```python
from build123d import *

# Parameters (mm, degrees)
SKETCH_1_W             = 60
SKETCH_1_H             = 124
EXTRUDE_1_DEPTH        = 3
EXTRUDE_2_DEPTH        = 3
SKETCH_3_W             = 136
SKETCH_3_H             = 57.699964
EXTRUDE_3_DEPTH        = 3
CUT_EXTRUDE_1_DEPTH    = 3
SKETCH_5_W             = 22
SKETCH_5_H             = 12
CUT_EXTRUDE_2_DEPTH    = 10
SKETCH_6_R             = 1.275
CUT_EXTRUDE_3_DEPTH    = 10
PATTERN_LINEAR_1_COUNT = 2
PATTERN_LINEAR_1_PITCH = 7.5
PATTERN_LINEAR_2_COUNT = 2
PATTERN_LINEAR_2_PITCH = 7.5
SKETCH_7_R             = 1.525
CUT_EXTRUDE_4_DEPTH    = 10
FILLET_1_R             = 2
SKETCH_8_W             = 21
SKETCH_8_H             = 41.4
CUT_EXTRUDE_5_DEPTH    = 22
FILLET_2_R             = 2
SKETCH_10_W            = 80
SKETCH_10_H            = 20.2
CUT_EXTRUDE_6_DEPTH    = 3
FILLET_3_R             = 2
CUT_EXTRUDE_7_DEPTH    = 3
EXTRUDE_5_DEPTH        = 3
CUT_EXTRUDE_START      = -22
SKETCH_13_R            = 5.6
CUT_EXTRUDE_8_DEPTH    = 115.070625066
FILLET_4_R             = 2


with BuildPart() as part:
    # 草图1 → 凸台-拉伸1 (new body)
    with BuildSketch(Plane.XY):
        Rectangle(SKETCH_1_W, SKETCH_1_H)
    extrude(amount=EXTRUDE_1_DEPTH)

    # 草图2 → 凸台-拉伸2 (add)
    with BuildSketch(Plane(origin=(0, 0, 0), x_dir=(-1, 0, 0), z_dir=(0, 0, -1))):
        Polygon((-66.648513504, -4.300036), (66.648513504, -4.300036), (30, 36.746299124), (-30, 36.746299124), align=None)
    extrude(amount=-EXTRUDE_2_DEPTH)

    # 草图3 → 凸台-拉伸3 (add)
    with BuildSketch(Plane.XY.offset(3)):
        with Locations((0, -33.150018)):
            Rectangle(SKETCH_3_W, SKETCH_3_H)
    extrude(amount=-EXTRUDE_3_DEPTH)

    # 草图4 → 切除-拉伸1 (cut)
    with BuildSketch(Plane.XY.offset(3)):
        Polygon((68, -4.300036), (68, -5.813700876), (66.648513504, -4.300036), align=None)
        Polygon((-66.648513504, -4.300036), (-68, -4.300036), (-68, -5.813700876), align=None)
    extrude(amount=-CUT_EXTRUDE_1_DEPTH, mode=Mode.SUBTRACT)

    # 草图5 → 切除-拉伸2 (cut)
    with BuildSketch(Plane(origin=(0, 0, 0), x_dir=(-1, 0, 0), z_dir=(0, 0, -1))):
        with Locations((-57, -56)):
            Rectangle(SKETCH_5_W, SKETCH_5_H)
    cut_extrude_2 = extrude(amount=-CUT_EXTRUDE_2_DEPTH, mode=Mode.SUBTRACT)

    # 镜向1: 切除-拉伸2 across plane
    add(cut_extrude_2.mirror(Plane(origin=(0, 0, 0), x_dir=(0, 0, 1), z_dir=(1, 0, 0))), mode=Mode.SUBTRACT)

    # 草图6 → 切除-拉伸3 (cut)
    with BuildSketch(Plane(origin=(0, 0, 0), x_dir=(-1, 0, 0), z_dir=(0, 0, -1))):
        with Locations((-27, 50.7)):
            Circle(SKETCH_6_R)
        with Locations((27, 50.7)):
            Circle(SKETCH_6_R)
        with Locations((27, -21.3)):
            Circle(SKETCH_6_R)
        with Locations((-27, -21.3)):
            Circle(SKETCH_6_R)
    cut_extrude_3 = extrude(amount=-CUT_EXTRUDE_3_DEPTH, mode=Mode.SUBTRACT)

    # 阵列(线性)1: 切除-拉伸3 ×2
    with Locations(*[(0, i * PATTERN_LINEAR_1_PITCH, 0) for i in range(1, PATTERN_LINEAR_1_COUNT)]):
        add(cut_extrude_3, mode=Mode.SUBTRACT)

    # 阵列(线性)2: 切除-拉伸3 ×2
    with Locations(*[(0, -i * PATTERN_LINEAR_2_PITCH, 0) for i in range(1, PATTERN_LINEAR_2_COUNT)]):
        add(cut_extrude_3, mode=Mode.SUBTRACT)

    # 草图7 → 切除-拉伸4 (cut)
    with BuildSketch(Plane(origin=(0, 0, 0), x_dir=(-1, 0, 0), z_dir=(0, 0, -1))):
        with Locations((65, -45)):
            Circle(SKETCH_7_R)
        with Locations((65, -25)):
            Circle(SKETCH_7_R)
        with Locations((41.234077164, 19.659734849)):
            Circle(SKETCH_7_R)
        with Locations((54.554392551, 4.740981616)):
            Circle(SKETCH_7_R)
    cut_extrude_4 = extrude(amount=-CUT_EXTRUDE_4_DEPTH, mode=Mode.SUBTRACT)

    # 镜向2: 切除-拉伸4 across plane
    add(cut_extrude_4.mirror(Plane(origin=(0, 0, 0), x_dir=(0, 0, 1), z_dir=(1, 0, 0))), mode=Mode.SUBTRACT)

    # 圆角1
    fillet_1_edges = [part.edges().sort_by_distance(p)[0] for p in [
        (-68, -50, 1.5),
        (-46, -62, 1.5),
        (-46, -50, 1.5),
        (-30, 36.746299124, 1.5),
        (30, 36.746299124, 1.5),
        (68, -5.813700876, 1.5),
        (-68, -5.813700876, 1.5),
        (-30, 62, 1.5),
        (30, 62, 1.5),
        (68, -50, 1.5),
        (46, -50, 1.5),
        (46, -62, 1.5),
    ]]
    fillet(fillet_1_edges, radius=FILLET_1_R)

    # 草图8 → 切除-拉伸5 (cut)
    with BuildSketch(Plane(origin=(0, 0, 0), x_dir=(-1, 0, 0), z_dir=(0, 0, -1))):
        with Locations((-13.5, -11.1)):
            Rectangle(SKETCH_8_W, SKETCH_8_H)
        with Locations((13.5, -11.1)):
            Rectangle(SKETCH_8_W, SKETCH_8_H)
        with Locations((13.5, 36.3)):
            Rectangle(SKETCH_8_W, SKETCH_8_H)
        with Locations((-13.5, 36.3)):
            Rectangle(SKETCH_8_W, SKETCH_8_H)
    extrude(amount=-CUT_EXTRUDE_5_DEPTH, mode=Mode.SUBTRACT)

    # 圆角2
    fillet_2_edges = [part.edges().sort_by_distance(p)[0] for p in [
        (24, 15.6, 1.5),
        (24, 57, 1.5),
        (3, 57, 1.5),
        (3, 15.6, 1.5),
        (-3, 57, 1.5),
        (-24, 57, 1.5),
        (-24, 15.6, 1.5),
        (-3, 15.6, 1.5),
        (-3, 9.6, 1.5),
        (-24, 9.6, 1.5),
        (-24, -31.8, 1.5),
        (-3, -31.8, 1.5),
        (3, 9.6, 1.5),
        (3, -31.8, 1.5),
        (24, -31.8, 1.5),
        (24, 9.6, 1.5),
    ]]
    fillet(fillet_2_edges, radius=FILLET_2_R)

    # 草图10 → 切除-拉伸6 (cut)
    with BuildSketch(Plane(origin=(0, 0, 0), x_dir=(-1, 0, 0), z_dir=(0, 0, -1))):
        with Locations((0, -46.9)):
            Rectangle(SKETCH_10_W, SKETCH_10_H)
    extrude(amount=-CUT_EXTRUDE_6_DEPTH, mode=Mode.SUBTRACT)

    # 圆角3
    fillet_3_edges = [part.edges().sort_by_distance(p)[0] for p in [
        (-40, -36.8, 1.5),
        (-40, -57, 1.5),
        (40, -57, 1.5),
        (40, -36.8, 1.5),
    ]]
    fillet(fillet_3_edges, radius=FILLET_3_R)

    # 草图11 → 切除-拉伸7 (cut)
    with BuildSketch(Plane.XY.offset(3)):
        Polygon((-31, 26.617503422), (-59, -4.742496578), (-59, -30.8), (-31, -30.8), align=None)
    cut_extrude_7 = extrude(amount=-CUT_EXTRUDE_7_DEPTH, mode=Mode.SUBTRACT)

    # 镜向3: 切除-拉伸7 across plane
    add(cut_extrude_7.mirror(Plane(origin=(0, 0, 0), x_dir=(0, 0, 1), z_dir=(1, 0, 0))), mode=Mode.SUBTRACT)

    # 草图12 → 凸台-拉伸5 (add)
    with BuildSketch(Plane(origin=(0, 0, 0), x_dir=(-1, 0, 0), z_dir=(0, 0, -1))):
        with BuildLine():
            Line((-59, -6.742496578), (-31, -6.742496578))
            ThreePointArc((-31, -6.742496578), (-29, -4.742496578), (-31, -2.742496578))
            Line((-31, -2.742496578), (-59, -2.742496578))
            ThreePointArc((-59, -2.742496578), (-61, -4.742496578), (-59, -6.742496578))
        make_face()
    extrude_5 = extrude(amount=-EXTRUDE_5_DEPTH)

    # 镜向4: 凸台-拉伸5 across plane
    add(extrude_5.mirror(Plane(origin=(0, 0, 0), x_dir=(0, 0, 1), z_dir=(1, 0, 0))))

    # 草图13 → 切除-拉伸8 (cut)
    with BuildSketch(Plane(origin=(0, 0, 0), x_dir=(-1, 0, 0), z_dir=(0, 0, -1)).offset(CUT_EXTRUDE_START)):
        with Locations(Location((53.4, -40.4, 0), (0, 0, 180))):
            Circle(SKETCH_13_R)
    cut_extrude_8 = extrude(amount=CUT_EXTRUDE_8_DEPTH, mode=Mode.SUBTRACT)

    # 镜向5: 切除-拉伸8 across plane
    add(cut_extrude_8.mirror(Plane(origin=(0, 0, 0), x_dir=(0, 0, 1), z_dir=(1, 0, 0))), mode=Mode.SUBTRACT)

    # 圆角4
    fillet_4_edges = [part.edges().sort_by_distance(p)[0] for p in [
        (-59, -30.8, 1.5),
        (-31, -30.8, 1.5),
        (-31, 26.617503422, 1.5),
        (31, -30.8, 1.5),
        (31, 26.617503422, 1.5),
        (59, -30.8, 1.5),
        (57.214285714, -2.742496578, 1.5),
        (59, -6.742496578, 1.5),
        (31, -2.742496578, 1.5),
        (31, -6.742496578, 1.5),
        (-57.214285714, -2.742496578, 1.5),
        (-31, -2.742496578, 1.5),
        (-31, -6.742496578, 1.5),
        (-59, -6.742496578, 1.5),
    ]]
    fillet(fillet_4_edges, radius=FILLET_4_R)


solid = part.part
```
Read the model definition and answer for the solid it produces. Units are mm, in the model's axes. A direction names the side the tool comes from. Coordinates: 2 decimals unless noted, no trailing zeros. Write each loop counter-clockwise with the first axis right and the second up, starting at its lowest first coordinate (ties: lowest second). Pieces come first, ordered by that corner, then holes. Notation, with made-up numbers: (37, 62) - (92, 62) arc R27 ccw to (92, 91) - close; hole circle Ø1 at (55.5, 81.5). An arc over 180 degrees is marked (long way). Answer as a JSON object with one key per item and string values. Group by question number.
1. A cutting plane is placed at B-B (x = 19.5). Determine the outline of the cut face in (y, z), plus the area to 3 significant figures.
2. Consider L1, parallel to X at y = -11, z = 1.35; L2, parallel to Y at x = 9.5, z = 1.4; L3, parallel to X at y = -56, z = 2.4. Determine where each line is inside the solid, lowest interval first. Write a range as [from, to].
3. A cutting plane is placed at C-C (x = -51). Determine the outline of the cut face in (y, z).
4. A cutting plane is placed at D-D (z = 1.95). Give the number of separate pieces and of enclosed holes in the cut face, plus the area to 3 significant figures.
5. Which of the six approach directions +Z, -Z, +X, -X, +Y, -Y give full straight-line access (tool end or side, diameter ignored) to faces 5 (the flat face through (0, 62, 1)), 6 (the flat face through (-3, -11, 1)), 7 (the flat face through (-30, 49, 1))?
6. Each of these flat-tipped pins is pushed along its axis until it touches: P1, Ø1.5, axis at x = 58.5, z = 1, coming from the -Y side; P2, Ø1, axis at y = -1, z = 1.5, coming from the +X side; P3, Ø1.5, axis at x = 46, z = 1.5, coming from the +Y side. Where does it stop, or does it pass through?
7. A cutting plane is placed at A-A (y = -25). Determine the outline of the cut face in (x, z) (3 decimals), plus the area to 3 significant figures.
8. The mould has two halves that part along Y. Classify faces 1 (the flat face through (-57, -50, 1)), 2 (the flat face through (24, 36, 1)), 3 (the flat face through (-1, 1, 3)), 4 (the flat face through (14, 57, 1)): +Y half, -Y half, draft (parallel to the pull), parting line (faces both ways), or undercut.
Worked out:
{
 "1": {"outline": "(-62, 0) - (-57, 0) - (-57, 3) - (-62, 3) - close; (-36.8, 0) - (-31.8, 0) - (-31.8, 3) - (-36.8, 3) - close; (9.6, 0) - (15.6, 0) - (15.6, 3) - (9.6, 3) - close; (57, 0) - (62, 0) - (62, 3) - (57, 3) - close", "area": "63.0 mm²"},
 "2": {"L1": "x = [-68, -59], [-31, -24], [-3, 3], [24, 31], [59, 68]", "L2": "y = [-62, -57], [-36.8, -31.8], [9.6, 15.6], [57, 62]", "L3": "x = [-46, -39.73], [39.73, 46]"},
 "3": {"outline": "(-50, 0) - (-45.46, 0) - (-45.46, 3) - (-50, 3) - close; (-35.34, 0) - (-30.8, 0) - (-30.8, 3) - (-35.34, 3) - close; (-6.74, 0) - (-2.74, 0) - (-2.74, 3) - (-6.74, 3) - close; (4.22, 0) - (13.23, 0) - (13.23, 3) - (4.22, 3) - close"},
 "4": {"separate pieces": "1", "enclosed holes": "31", "area": "5,310 mm²"},
 "5": {"face 5": "+Z, -Z, +X, -X, +Y", "face 6": "+Z, -Z", "face 7": "+Z, -Z, -X, +Y"},
 "6": {"P1": "stops at y = -50", "P2": "stops at x = 64.15", "P3": "stops at y = 19.67"},
 "7": {"outline": "(-68, 0) - (-66.525, 0) - (-66.525, 3) - (-68, 3) - close; (-63.475, 0) - (-59, 0) - (-59, 3) - (-63.475, 3) - close; (-31, 0) - (-24, 0) - (-24, 3) - (-31, 3) - close; (-3, 0) - (3, 0) - (3, 3) - (-3, 3) - close; (24, 0) - (31, 0) - (31, 3) - (24, 3) - close; (59, 0) - (63.475, 0) - (63.475, 3) - (59, 3) - close; (66.525, 0) - (68, 0) - (68, 3) - (66.525, 3) - close", "area": "95.7 mm²"},
 "8": {"face 1": "-Y half", "face 2": "undercut", "face 3": "draft", "face 4": "undercut"}
}
